For this review, use the dimensioned drawing (mm, ordinates from the lowest corner) and the shaded views. A direction names the side the tool comes from. Coordinates: 2 decimals unless noted, no trailing zeros. Loops run counter-clockwise (first coordinate to the right, second up) from the corner with the lowest first, then second, coordinate; pieces in that order, holes last. Notation, with made-up numbers: (-26, 75.5) -> (-5, 75.5) arc R15 cw to (-5, 84.5) -> close; hole circle Ø1 at (67, 70.25). An arc over 180 degrees is marked (long way). Answer as a JSON object with one key per item and string values.
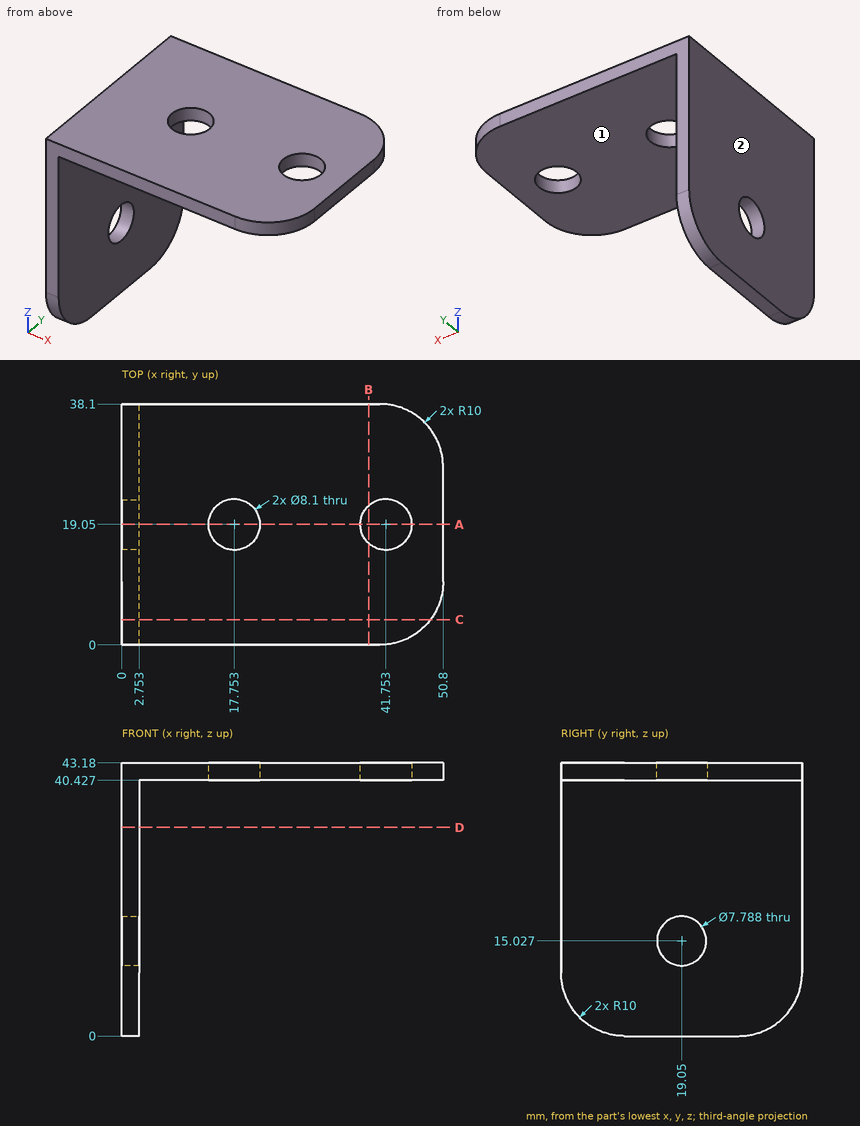
1) For the marked faces 1 and 2, list the 3-axis set-ups (+Z, -Z, +X, -X, +Y, -Y) from which the entire face can be reached by the end or side of a thin tool; tool diameter is ignored.
Completed:
{"face 1": "-Z, +X, +Y, -Y", "face 2": "+Z, -Z, -X, +Y, -Y"}
2) Wall thickness on probe 1 along X at (y, z) = (19, 41); probe 2 along X at (y, z) = (4, 39); probe 3 along Z at (x, y) = (12.5, 14.5): over which ranges is each line inside the solid? List them lowest first.
Completed:
{"probe 1": "0 to 13.7, 21.8 to 37.7, 45.8 to 50.8", "probe 2": "0 to 2.75", "probe 3": "40.43 to 43.18"}
3) Add section D-D, the plane z = 33. Give the boundary of the cut face in (x, y), and give its area (3 significant figures).
Completed:
{"outline": "(0, 0) -> (2.75, 0) -> (2.75, 38.1) -> (0, 38.1) -> close", "area": "105 mm²"}
4) Clearance check with flat-ended pins moving along their axes: pin 1 Ø9.5 at (x, y) = (17.75, 19.05) entering from -Z; pin 2 Ø11.5 at (y, z) = (18.5, 12) entering from +X; pin 3 Ø10 at (y, z) = (4, 36) entering from +X. State where each tip first meets the part, or that it passes through.
Completed:
{"pin 1": "z = 40.43", "pin 2": "x = 2.75", "pin 3": "x = 50.1"}
5) Add section B-B, the plane x = 39. Give the boundary of the cut face in (y, z).
Completed:
{"outline": "(0, 40.43) -> (16.08, 40.43) -> (16.08, 43.18) -> (0, 43.18) -> close; (22.02, 40.43) -> (38.1, 40.43) -> (38.1, 43.18) -> (22.02, 43.18) -> close"}
6) Add section A-A, the plane y = 19.05. Give the boundary of the cut face in (x, z), and give its area (3 significant figures).
Completed:
{"outline": "(0, 0) -> (2.75, 0) -> (2.75, 11.13) -> (0, 11.13) -> close; (0, 18.92) -> (2.75, 18.92) -> (2.75, 40.43) -> (13.7, 40.43) -> (13.7, 43.18) -> (0, 43.18) -> close; (21.8, 40.43) -> (37.7, 40.43) -> (37.7, 43.18) -> (21.8, 43.18) -> close; (45.8, 40.43) -> (50.8, 40.43) -> (50.8, 43.18) -> (45.8, 43.18) -> close", "area": "185 mm²"}
7) Add section C-C, the plane y = 4. Give the boundary of the cut face in (x, z), and give its area (3 significant figures).
Completed:
{"outline": "(0, 2) -> (2.75, 2) -> (2.75, 40.43) -> (48.8, 40.43) -> (48.8, 43.18) -> (0, 43.18) -> close", "area": "240 mm²"}
